The figure shows three views and two pictorial views of one solid part (mm, origin at its lowest corner). Answer the questions. Round coordinates to 2 decimals unless told otherwise and drop trailing zeros. Order: outer loops, then holes, each group sorted by start corner. A loop starts at its lowest first (then second) coordinate and runs counter-clockwise, first axis right, second up. Notation, with made-up numbers: (18, 5) -> (47, 5) arc R15 cw to (47, 17) -> close; hole circle Ø3 at (11, 21). An arc over 180 degrees is marked (long way). Return JSON: item names as keys, results as strings. Group by question number.
(1) Consider line 1 (Y direction, x = 30, z = 5.75); line 2 (Y direction, x = 21, z = 1.25); line 3 (Z direction, x = 37, y = 55.5). Determine where each line is inside the solid, lowest interval first. Write a range as [from, to].
(2) The part is cut by section B-B (y = 30). Determine the outline of the cut face in (x, z), plus the area to 3 significant figures.
(3) The part is cut by section D-D (z = 2.75). Count the separate pieces of the cut face and the enclosed holes in it, plus the area to 3 significant figures.
(4) Determine the mould class of the marked faces 1, 2 and 3 for opening direction X: +X half, -X half, draft (parallel to the pull), parting line (faces both ways), or undercut.
(5) Each of these flat-tipped pins is pushed along its axis until it touches: pin 1 (1.5 mm diameter, centred on x = 45.5, z = 5, fed in from -Y); pin 2 (2.5 mm diameter, centred on x = 20.91, y = 35.25, fed in from -Z); pin 3 (1.5 mm diameter, centred on y = 48, z = 3, fed in from -X); pin 4 (5 mm diameter, centred on x = 53.5, z = 6.5, fed in from -Y) (1 decimal). Where does it stop, or does it pass through?
(6) The part is cut by section C-C (z = 8.5). Determine the outline of the cut face in (x, y), plus the area to 3 significant figures.
(7) The part is cut by section A-A (x = 30). Determine the outline of the cut face in (y, z), plus the area to 3 significant figures.
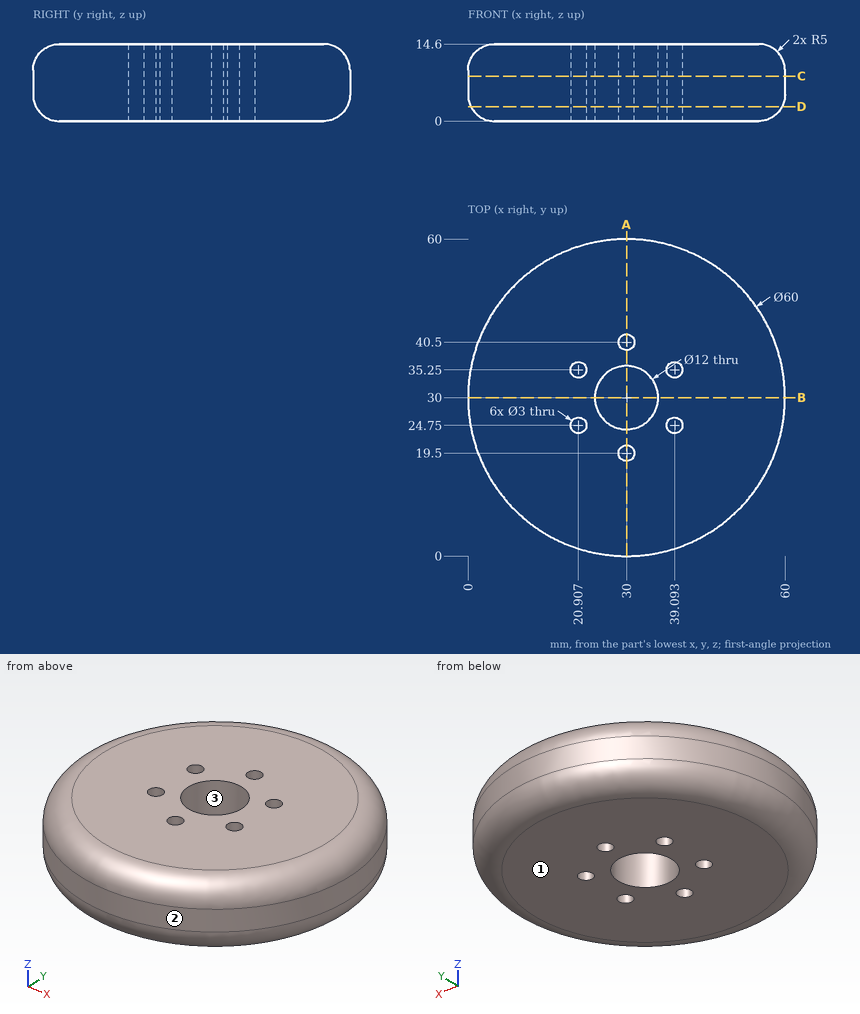
Answer below:
{
 "1": {"line 1": "y = [0, 18], [21, 24], [36, 39], [42, 60]", "line 2": "y = [3.16, 23.25], [26.25, 33.75], [36.75, 56.84]", "line 3": "z = [0.21, 14.39]"},
 "2": {"outline": "(0, 5) arc R5 ccw to (5, 0) -> (24, 0) -> (24, 14.6) -> (5, 14.6) arc R5 ccw to (0, 9.6) -> close; (36, 0) -> (55, 0) arc R5 ccw to (60, 5) -> (60, 9.6) arc R5 ccw to (55, 14.6) -> (36, 14.6) -> close", "area": "679 mm²"},
 "3": {"separate pieces": "1", "enclosed holes": "7", "area": "2,570 mm²"},
 "4": {"face 1": "draft", "face 2": "parting line", "face 3": "undercut"},
 "5": {"pin 1": "stops at y = 3.88", "pin 2": "passes through", "pin 3": "stops at x = 5.86", "pin 4": "stops at y = 8.6"},
 "6": {"outline": "circle Ø60 at (30, 30); hole circle Ø3 at (20.91, 24.75); hole circle Ø3 at (20.91, 35.25); hole circle Ø12 at (30, 30); hole circle Ø3 at (30, 19.5); hole circle Ø3 at (30, 40.5); hole circle Ø3 at (39.09, 24.75); hole circle Ø3 at (39.09, 35.25)", "area": "2,670 mm²"},
 "7": {"outline": "(0, 5) arc R5 ccw to (5, 0) -> (18, 0) -> (18, 14.6) -> (5, 14.6) arc R5 ccw to (0, 9.6) -> close; (21, 0) -> (24, 0) -> (24, 14.6) -> (21, 14.6) -> close; (36, 0) -> (39, 0) -> (39, 14.6) -> (36, 14.6) -> close; (42, 0) -> (55, 0) arc R5 ccw to (60, 5) -> (60, 9.6) arc R5 ccw to (55, 14.6) -> (42, 14.6) -> close", "area": "592 mm²"}
}
